```python
from build123d import *

# Parameters (mm, degrees)
F0_R     = 5
F0_R_2   = 2.3
F1_DEPTH = 5
F2_START = 5
F2_DEPTH = 1
F3_START = 6
F3_DEPTH = 130
F4_START = 136
F4_DEPTH = 1
F5_START = 137
F5_DEPTH = 5
F6_SIZE  = 1.8


with BuildPart() as f1:
    # F0 (on Top) → F1 (new body)
    with BuildSketch(Plane.XY):
        Circle(F0_R)
        Circle(F0_R_2, mode=Mode.SUBTRACT)
        Circle(F0_R_2)
    extrude(amount=F1_DEPTH)

    # F0 (on Top) → F2 (join)
    with BuildSketch(Plane.XY.offset(F2_START)):
        Circle(F0_R_2)
    extrude(amount=F2_DEPTH)

    # F0 (on Top) → F3 (join)
    with BuildSketch(Plane.XY.offset(F3_START)):
        Circle(F0_R)
        Circle(F0_R_2, mode=Mode.SUBTRACT)
        Circle(F0_R_2)
    extrude(amount=F3_DEPTH)

    # F0 (on Top) → F4 (join)
    with BuildSketch(Plane.XY.offset(F4_START)):
        Circle(F0_R_2)
    extrude(amount=F4_DEPTH)

    # F0 (on Top) → F5 (join)
    with BuildSketch(Plane.XY.offset(F5_START)):
        Circle(F0_R)
        Circle(F0_R_2, mode=Mode.SUBTRACT)
        Circle(F0_R_2)
    extrude(amount=F5_DEPTH)

    # F6
    f6_edges = [f1.edges().sort_by_distance(p)[0] for p in [
        (-5, 0, 136),
        (-5, 0, 137),
        (-5, 0, 6),
        (-5, 0, 5),
    ]]
    chamfer(f6_edges, length=F6_SIZE)


solid = f1.part
```
Input: part model. Units: mm. Frame: model coordinates. A direction names the side the tool comes from. Give positions to 0.01 mm unless a question says otherwise; leave off trailing zeros. Order: outer loops, then holes, each group sorted by start corner. A loop starts at its lowest first (then second) coordinate and runs counter-clockwise, first axis right, second up. Notation, with made-up numbers: (67.5, 2) - (87.5, 2) arc R14 cw to (87.5, 19) - close; hole circle Ø4 at (82.5, 55). An arc over 180 degrees is marked (long way). Put each result on its own line as item: value.
Item 1: Draft query along Z for faces 3 (the flat face through (0, 0, 142)), 4 (the cylindrical face through (-1.08, -4.88, 1.58)), 5 (the flat face through (2.1, -1.4, 136)). Return one class per face: +Z half, -Z half, draft (parallel to the pull), parting line (faces both ways), or undercut.
Found:
face 3: +Z half
face 4: draft
face 5: undercut
Item 2: Contact query for flat-ended pins moving along their axis: pin 1 (1 mm diameter, centred on x = 1, z = 35.5, fed in from +Y); pin 2 (1 mm diameter, centred on y = -2, z = 100, fed in from +X); pin 3 (1 mm diameter, centred on y = 1.5, z = 17, fed in from +X). Output: stop coordinate, or through.
Found:
pin 1: stops at y = 4.97
pin 2: stops at x = 4.77
pin 3: stops at x = 4.9
Item 3: Section query A-A, the plane y = 0. Return loops of the section in (x, z).
Found:
outline: (-5, 0) - (5, 0) - (5, 3.2) - (3.2, 5) - (2.3, 5) - (2.3, 6) - (3.2, 6) - (5, 7.8) - (5, 134.2) - (3.2, 136) - (2.3, 136) - (2.3, 137) - (3.2, 137) - (5, 138.8) - (5, 142) - (-5, 142) - (-5, 138.8) - (-3.2, 137) - (-2.3, 137) - (-2.3, 136) - (-3.2, 136) - (-5, 134.2) - (-5, 7.8) - (-3.2, 6) - (-2.3, 6) - (-2.3, 5) - (-3.2, 5) - (-5, 3.2) - close
Item 4: Access query for faces 1 (the conical face through (-0.72, -3.23, 135.89)), 2 (the cylindrical face through (-1.08, -4.88, 140.38)). Directions: +Z, -Z, +X, -X, +Y, -Y. A direction counts if a zero-diameter tool reaches every point of the face in a straight line with its end or side. Return the directions, or none.
Found:
face 1: none
face 2: +Z, -Z
Item 5: Ray query, L1, parallel to Z at x = -2.25, y = 4; L2, parallel to Z at x = 2.5, y = -3.25; L3, parallel to X at y = -0.5, z = 73.5. Return the intervals inside material, ascending. Write a range as from..to.
Found:
L1: z = 0..3.61, 7.39..134.61, 138.39..142
L2: z = 0..4.1, 6.9..135.1, 137.9..142
L3: x = -4.97..4.97
Item 6: Section query C-C, the plane z = 35. Return loops of the section in (x, y).
Found:
outline: circle Ø10 at (0, 0)
